```python
from build123d import *

# Parameters (mm, degrees)
F1_DEPTH = 2168
F4_R     = 4.5
F5_DEPTH = 4


with BuildPart() as f1:
    # F0 (on Front) → F1 (new body)
    with BuildSketch(Plane.XZ):
        with BuildLine():
            Line((-37.5, -42.25), (-37.5, -46.25))
            Line((-37.5, -46.25), (29.5, -46.25))
            ThreePointArc((29.5, -46.25), (35.1568542495, -43.9068542495), (37.5, -38.25))
            Line((37.5, -38.25), (37.5, 38.25))
            ThreePointArc((37.5, 38.25), (35.1568542495, 43.9068542495), (29.5, 46.25))
            Line((29.5, 46.25), (-37.5, 46.25))
            Line((-37.5, 46.25), (-37.5, 42.25))
            Line((-37.5, 42.25), (29.5, 42.25))
            ThreePointArc((29.5, 42.25), (32.3284271247, 41.0784271247), (33.5, 38.25))
            Line((33.5, 38.25), (33.5, -38.25))
            ThreePointArc((33.5, -38.25), (32.3284271247, -41.0784271247), (29.5, -42.25))
            Line((29.5, -42.25), (-37.5, -42.25))
        make_face()
    extrude(amount=-F1_DEPTH)

    # F4 (on offset) → F5 (cut, through all)
    with BuildSketch(Plane.XY.offset(46.25)):
        with BuildLine():
            ThreePointArc((15.867, 98), (11.367, 102.5), (6.867, 98))
            ThreePointArc((6.867, 98), (11.367, 93.5), (15.867, 98))
        make_face()
        with Locations((-20.2620720863, 129)):
            Circle(F4_R)
    extrude(amount=-F5_DEPTH, mode=Mode.SUBTRACT)


with BuildPart() as f7_1:
    # F7: instance of F1
    add(f1.part.mirror(Plane.YZ.offset(-250)))


solid = f7_1.part
```
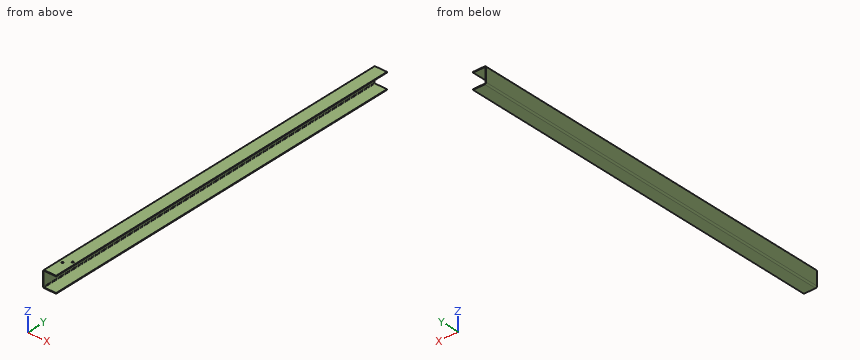
For this review, take the finished solid that the model builds, in its own axes (mm). Coordinates: 2 decimals unless noted, no trailing zeros. Loops run counter-clockwise (first coordinate to the right, second up) from the corner with the lowest first, then second, coordinate; pieces in that order, holes last. Notation, with made-up numbers: (52.25, 42) - (106.25, 42) arc R17 ccw to (106.25, 46) - close; hole circle Ø10 at (73, 87). An arc over 180 degrees is marked (long way). Use one line per item in the form item = value. Start each with the question number.
1) Take a section at B-B (z = -5). State the section outline as (x, y) points, plus the area to 3 significant figures.
2) To check wall thickness, follow probe 1 along Z at (x, y) = (-467.5, 1044.5); probe 2 along X at (y, z) = (98, 45); probe 3 along X at (y, z) = (1314.5, -30). State the ranges of each line that lie inside material, in increasing order. Write a range as from..to.
3) Take a section at A-A (y = 1952). State the section outline as (x, z) points.
From the geometry:
q1.outline = (-537.5, 0) - (-533.5, 0) - (-533.5, 2168) - (-537.5, 2168) - close
q1.area = 8,670 mm2
q2.probe_1 = -46.25..-42.25, 42.25..46.25
q2.probe_2 = -533.79..-515.87, -506.87..-462.5
q2.probe_3 = -537.5..-533.5
q3.outline = (-537.5, -38.25) arc R8 ccw to (-529.5, -46.25) - (-462.5, -46.25) - (-462.5, -42.25) - (-529.5, -42.25) arc R4 cw to (-533.5, -38.25) - (-533.5, 38.25) arc R4 cw to (-529.5, 42.25) - (-462.5, 42.25) - (-462.5, 46.25) - (-529.5, 46.25) arc R8 ccw to (-537.5, 38.25) - close
